Build history of the part. All positions in model axes, mm. A direction names the side the tool comes from. Round coordinates to 2 decimals unless told otherwise and drop trailing zeros. Write each loop counter-clockwise with the first axis right and the second up, starting at its lowest first coordinate (ties: lowest second). Pieces come first, ordered by that corner, then holes. Notation, with made-up numbers: (33.25, 28.5) -> (81.25, 28.5) arc R19 ccw to (81.25, 63.5) -> close; hole circle Ø10 at (70, -18.5). An arc over 180 degrees is marked (long way). Answer in a Markdown table with one row per item.
```python
from build123d import *

# Parameters (mm, degrees)
SKETCH_1_W                                   = 162
SKETCH_1_H                                   = 162
SKETCH_1_W_2                                 = 146
SKETCH_1_H_2                                 = 146
EXTRUDE_375_DEPTH                            = 7
SKETCH_2_W                                   = 10
SKETCH_2_H                                   = 3
EXTRUDE_670_DEPTH                            = 2
PATTERN_CIRCULAR_761_COUNT                   = 4
PATTERN_CIRCULAR_761_COPY_1_SKETCH_W         = 10
PATTERN_CIRCULAR_761_COPY_1_SKETCH_H         = 3
PATTERN_CIRCULAR_761_COPY_1_DEPTH            = 2
PATTERN_CIRCULAR_761_COPY_2_SKETCH_W         = 10
PATTERN_CIRCULAR_761_COPY_2_SKETCH_H         = 3
PATTERN_CIRCULAR_761_COPY_2_DEPTH            = 2
PATTERN_CIRCULAR_761_COPY_3_SKETCH_W         = 10
PATTERN_CIRCULAR_761_COPY_3_SKETCH_H         = 3
PATTERN_CIRCULAR_761_COPY_3_DEPTH            = 2
SKETCH_3_R                                   = 1.7
CUT_EXTRUDE_1047_DEPTH                       = 115.764977236
MIRROR_1214_COPY_1_SKETCH_R                  = 1.7
MIRROR_1214_COPY_1_DEPTH                     = 115.764977236
SKETCH_4_R                                   = 1.65
CUT_EXTRUDE_1505_DEPTH                       = 3.5
MIRROR_1637_COPY_1_SKETCH_R                  = 1.65
MIRROR_1637_COPY_1_DEPTH                     = 3.5
CUT_EXTRUDE_2611_DEPTH                       = 2.6
MIRROR_2701_AT_THE_SECOND_PLANE_COPY_1_DEPTH = 2.6
FILLET_1_R                                   = 0.5
FILLET_2_R                                   = 0.5


with BuildPart() as part:
    # Эскиз1 → Extrude 375 (new body)
    with BuildSketch(Plane.XY):
        Rectangle(SKETCH_1_W, SKETCH_1_H)
        Rectangle(SKETCH_1_W_2, SKETCH_1_H_2, mode=Mode.SUBTRACT)
    extrude(amount=EXTRUDE_375_DEPTH)

    # Эскиз2 → Extrude 670 (add)
    with BuildSketch(Plane(origin=(0, 0, 0), x_dir=(-1, 0, 0), z_dir=(0, 0, -1))):
        with Locations((-38, 72.5)):
            Rectangle(SKETCH_2_W, SKETCH_2_H)
    extrude_670 = extrude(amount=-EXTRUDE_670_DEPTH)

    # Mirror 726: Extrude 670 across plane
    add(extrude_670.mirror(Plane(origin=(0, 0, 0), x_dir=(0, 0, 1), z_dir=(1, 0, 0))))

    # Pattern Circular 761: Extrude 670 ×4 about axis
    pattern_circular_761_axis = Axis((0, 0, 0), (0, 0, 1))
    for i in range(1, PATTERN_CIRCULAR_761_COUNT):
        add(extrude_670.rotate(pattern_circular_761_axis, i * 360 / PATTERN_CIRCULAR_761_COUNT))

    # Pattern Circular 761 copy 1 sketch → Pattern Circular 761 copy 1 (add)
    with BuildSketch(Plane.YX):
        with Locations((-38, -72.5)):
            Rectangle(PATTERN_CIRCULAR_761_COPY_1_SKETCH_W, PATTERN_CIRCULAR_761_COPY_1_SKETCH_H)
    extrude(amount=-PATTERN_CIRCULAR_761_COPY_1_DEPTH)

    # Pattern Circular 761 copy 2 sketch → Pattern Circular 761 copy 2 (add)
    with BuildSketch(Plane(origin=(0, 0, 0), x_dir=(-1, 0, 0), z_dir=(0, 0, -1))):
        with Locations((-38, -72.5)):
            Rectangle(PATTERN_CIRCULAR_761_COPY_2_SKETCH_W, PATTERN_CIRCULAR_761_COPY_2_SKETCH_H)
    extrude(amount=-PATTERN_CIRCULAR_761_COPY_2_DEPTH)

    # Pattern Circular 761 copy 3 sketch → Pattern Circular 761 copy 3 (add)
    with BuildSketch(Plane(origin=(0, 0, 0), x_dir=(0, -1, 0), z_dir=(0, 0, -1))):
        with Locations((-38, -72.5)):
            Rectangle(PATTERN_CIRCULAR_761_COPY_3_SKETCH_W, PATTERN_CIRCULAR_761_COPY_3_SKETCH_H)
    extrude(amount=-PATTERN_CIRCULAR_761_COPY_3_DEPTH)

    # Эскиз3 → Cut-Extrude 1047 (cut, through all)
    with BuildSketch(Plane.XY.offset(7)):
        with Locations((-77, 77)):
            Circle(SKETCH_3_R)
    cut_extrude_1047 = extrude(amount=-CUT_EXTRUDE_1047_DEPTH, mode=Mode.SUBTRACT)

    # Mirror 1158: Cut-Extrude 1047 across plane
    add(cut_extrude_1047.mirror(Plane(origin=(0, 0, 0), x_dir=(0, 0, 1), z_dir=(1, 0, 0))), mode=Mode.SUBTRACT)

    # Mirror 1214: Cut-Extrude 1047 across plane
    add(cut_extrude_1047.mirror(Plane.ZX), mode=Mode.SUBTRACT)

    # Mirror 1214 copy 1 sketch → Mirror 1214 copy 1 (cut, through all)
    with BuildSketch(Plane(origin=(0, 0, 7), x_dir=(-1, 0, 0), z_dir=(0, 0, 1))):
        with Locations((-77, 77)):
            Circle(MIRROR_1214_COPY_1_SKETCH_R)
    extrude(amount=-MIRROR_1214_COPY_1_DEPTH, mode=Mode.SUBTRACT)

    # Эскиз4 → Cut-Extrude 1505 (cut)
    with BuildSketch(Plane.XY.offset(7)):
        with Locations((-77, 68)):
            Circle(SKETCH_4_R)
    cut_extrude_1505 = extrude(amount=-CUT_EXTRUDE_1505_DEPTH, mode=Mode.SUBTRACT)

    # Mirror 1581: Cut-Extrude 1505 across plane
    add(cut_extrude_1505.mirror(Plane(origin=(0, 0, 0), x_dir=(0, 0, 1), z_dir=(1, 0, 0))), mode=Mode.SUBTRACT)

    # Mirror 1637: Cut-Extrude 1505 across plane
    add(cut_extrude_1505.mirror(Plane.ZX), mode=Mode.SUBTRACT)

    # Mirror 1637 copy 1 sketch → Mirror 1637 copy 1 (cut)
    with BuildSketch(Plane(origin=(0, 0, 7), x_dir=(-1, 0, 0), z_dir=(0, 0, 1))):
        with Locations((-77, 68)):
            Circle(MIRROR_1637_COPY_1_SKETCH_R)
    extrude(amount=-MIRROR_1637_COPY_1_DEPTH, mode=Mode.SUBTRACT)

    # Эскиз5 → Cut-Extrude 2611 (cut)
    with BuildSketch(Plane(origin=(0, 0, 0), x_dir=(-1, 0, 0), z_dir=(0, 0, -1))):
        Polygon((-73.651368439, 77), (-75.325684219, 79.9), (-78.674315781, 79.9), (-80.348631561, 77), (-78.674315781, 74.1), (-75.325684219, 74.1), align=None)
    cut_extrude_2611 = extrude(amount=-CUT_EXTRUDE_2611_DEPTH, mode=Mode.SUBTRACT)

    # Mirror 2701: Cut-Extrude 2611 across plane
    add(cut_extrude_2611.mirror(Plane(origin=(0, 0, 0), x_dir=(0, 0, 1), z_dir=(1, 0, 0))), mode=Mode.SUBTRACT)

    # Mirror 2701 at the second plane: Cut-Extrude 2611 across plane
    add(cut_extrude_2611.mirror(Plane.ZX), mode=Mode.SUBTRACT)

    # Mirror 2701 at the second plane copy 1 s → Mirror 2701 at the second plane copy 1 (cut)
    with BuildSketch(Plane(origin=(0, 0, 0), x_dir=(1, 0, 0), z_dir=(0, 0, -1))):
        Polygon((-73.651368439, 77), (-75.325684219, 79.9), (-78.674315781, 79.9), (-80.348631561, 77), (-78.674315781, 74.1), (-75.325684219, 74.1), align=None)
    extrude(amount=-MIRROR_2701_AT_THE_SECOND_PLANE_COPY_1_DEPTH, mode=Mode.SUBTRACT)

    # Скругление1
    fillet_1_edges = [part.edges().sort_by_distance(p)[0] for p in [
        (0, -81, 0),
        (-81, 0, 0),
        (0, 81, 0),
        (81, 0, 0),
    ]]
    fillet(fillet_1_edges, radius=FILLET_1_R)

    # Скругление2
    # the kernel refuses this fillet: 0.5 mm, written as the material it takes off along each edge
    with BuildSketch(Plane(origin=(-80.5, 80.5, 0.5), x_dir=(-1, 0, 0), z_dir=(0, 1, 0))) as fillet_2_piece_1_section:
        Polygon((0, 0), (FILLET_2_R, 0), (FILLET_2_R, -FILLET_2_R), (0, -FILLET_2_R), align=None)
    fillet_2_piece_1 = extrude(amount=FILLET_2_R, mode=Mode.PRIVATE)
    fillet_2_piece_1 = fillet_2_piece_1 - Plane(origin=(-80.5, 80.5, 0.5), x_dir=(0.7071067811865475, 0, 0.7071067811865475), z_dir=(0, 1, 0)) * Sphere(FILLET_2_R, mode=Mode.PRIVATE)
    add(fillet_2_piece_1, mode=Mode.SUBTRACT)
    with BuildSketch(Plane(origin=(80.5, 80.5, 0.5), x_dir=(1, 0, 0), z_dir=(0, 1, 0))) as fillet_2_piece_2_section:
        Polygon((0, 0), (FILLET_2_R, 0), (FILLET_2_R, FILLET_2_R), (0, FILLET_2_R), align=None)
    fillet_2_piece_2 = extrude(amount=FILLET_2_R, mode=Mode.PRIVATE)
    fillet_2_piece_2 = fillet_2_piece_2 - Plane(origin=(80.5, 80.5, 0.5), x_dir=(-0.7071067811865475, 0, 0.7071067811865475), z_dir=(0, 1, 0)) * Sphere(FILLET_2_R, mode=Mode.PRIVATE)
    add(fillet_2_piece_2, mode=Mode.SUBTRACT)
    with BuildSketch(Plane(origin=(-80.5, -80.5, 0.5), x_dir=(0, -1, 0), z_dir=(-1, 0, 0))) as fillet_2_piece_3_section:
        Polygon((0, 0), (FILLET_2_R, 0), (FILLET_2_R, -FILLET_2_R), (0, -FILLET_2_R), align=None)
    fillet_2_piece_3 = extrude(amount=FILLET_2_R, mode=Mode.PRIVATE)
    fillet_2_piece_3 = fillet_2_piece_3 - Plane(origin=(-80.5, -80.5, 0.5), x_dir=(0, 0.7071067811865475, 0.7071067811865475), z_dir=(-1, 0, 0)) * Sphere(FILLET_2_R, mode=Mode.PRIVATE)
    add(fillet_2_piece_3, mode=Mode.SUBTRACT)
    with BuildSketch(Plane(origin=(80.5, -80.5, 0.5), x_dir=(0, -1, 0), z_dir=(1, 0, 0))) as fillet_2_piece_4_section:
        Polygon((0, 0), (FILLET_2_R, 0), (FILLET_2_R, FILLET_2_R), (0, FILLET_2_R), align=None)
    fillet_2_piece_4 = extrude(amount=FILLET_2_R, mode=Mode.PRIVATE)
    fillet_2_piece_4 = fillet_2_piece_4 - Plane(origin=(80.5, -80.5, 0.5), x_dir=(0, 0.7071067811865475, 0.7071067811865475), z_dir=(1, 0, 0)) * Sphere(FILLET_2_R, mode=Mode.PRIVATE)
    add(fillet_2_piece_4, mode=Mode.SUBTRACT)
    with BuildSketch(Plane(origin=(81, -81, 0.5), x_dir=(0, 1, 0), z_dir=(0, 0, 1)), Plane(origin=(81, 81, 0.5), x_dir=(-1, 0, 0), z_dir=(0, 0, 1))) as fillet_2_piece_5:
        with BuildLine():
            CenterArc((FILLET_2_R, FILLET_2_R), FILLET_2_R, 180, 90)
            Line((0, FILLET_2_R), (0, 0))
            Line((0, 0), (FILLET_2_R, 0))
        make_face()
    extrude(amount=7.75, mode=Mode.SUBTRACT)
    with BuildSketch(Plane(origin=(-81, -81, 0.5), x_dir=(0, 1, 0), z_dir=(0, 0, 1)), Plane(origin=(-81, 81, 0.5), x_dir=(1, 0, 0), z_dir=(0, 0, 1))) as fillet_2_piece_6:
        with BuildLine():
            CenterArc((FILLET_2_R, -FILLET_2_R), FILLET_2_R, 90, 90)
            Line((0, -FILLET_2_R), (0, 0))
            Line((0, 0), (FILLET_2_R, 0))
        make_face()
    extrude(amount=7.75, mode=Mode.SUBTRACT)


solid = part.part
```
Q1. Saw through at A-A on y = -35.5. Write the cut outline in (x, z), plus the area to 3 significant figures.
A:
| item | result |
|---|---|
| outline | (-81, 0.5) arc R0.5 ccw to (-80.5, 0) -> (-71, 0) -> (-71, 2) -> (-73, 2) -> (-73, 7) -> (-81, 7) -> close; (71, 0) -> (80.5, 0) arc R0.5 ccw to (81, 0.5) -> (81, 7) -> (73, 7) -> (73, 2) -> (71, 2) -> close |
| area | 120 mm² |
Q2. Drop a flat-ended pin along its axis: P1, Ø2, axis at x = 37.5, y = -71.5, coming from the +Z side. Give the stop position or say it passes through.
A:
| item | result |
|---|---|
| P1 | z = 2 |
Q3. Which spindle directions (+Z, -Z, +X, -X, +Y, -Y) get a long thin tool onto all of the face, cutting with end or side? Do faces 4 (the flat face through (75.6, 78.3, 2.6)), 5 (the flat face through (-78, 0, 7)). Say none if no direction does.
A:
| item | result |
|---|---|
| face 4 | -Z |
| face 5 | +Z, +X, -X, +Y, -Y |
Q4. Saw through at B-B on x = 67.5. Write the cut outline in (y, z).
A:
| item | result |
|---|---|
| outline | (-81, 0.5) arc R0.5 ccw to (-80.5, 0) -> (-73, 0) -> (-73, 7) -> (-81, 7) -> close; (73, 0) -> (80.5, 0) arc R0.5 ccw to (81, 0.5) -> (81, 7) -> (73, 7) -> close |
Q5. Wall check: line 1 (Y direction, x = 77, z = 5.6); line 2 (X direction, y = -77, z = 5.85); line 3 (Y direction, x = 62.5, z = 3.5). Give the ranges that are in metal, low to high. Write a range as [from, to].
A:
| item | result |
|---|---|
| line 1 | [-81, -78.7], [-75.3, -69.65], [-66.35, 66.35], [69.65, 75.3], [78.7, 81] |
| line 2 | [-81, -78.7], [-75.3, 75.3], [78.7, 81] |
| line 3 | [-81, -73], [73, 81] |
Q6. Two-plate mould, pull along Y, no slides. Class faces 1 (the flat face through (73, -1, 3)), 2 (the flat face through (78, 0, 0)), 3 (the flat face through (-1, 81, 4)): released by +Y, released by -Y, zero draft, split by the parting line, or undercut.
A:
| item | result |
|---|---|
| face 1 | undercut |
| face 2 | zero draft |
| face 3 | released by +Y |
